Design review of the part built by this model. Coordinates are the model's own, in mm. A direction names the side the tool comes from. Give positions to 0.01 mm unless a question says otherwise; leave off trailing zeros. Loops run counter-clockwise (first coordinate to the right, second up) from the corner with the lowest first, then second, coordinate; pieces in that order, holes last. Notation, with made-up numbers: (-17.75, -17.5) - (-1.75, -17.5) arc R11 cw to (-1.75, -7.5) - close; hole circle Ø4 at (75.5, 35). An arc over 180 degrees is marked (long way). Write each question's results on one line, items separated by ' | '.
from build123d import *

# Parameters (mm, degrees)
SCHIZZO1_R                                           = 273.53258218
ESTRUSIONE_ESTRUSIONE1_DEPTH                         = 15
SCHIZZO5_R                                           = 273.53258218
ESTRUSIONE_ESTRUSIONE4_DEPTH                         = 685
SCHIZZO6_R                                           = 350
ESTRUSIONE_ESTRUSIONE5_DEPTH                         = 30
SMUSSO2_SIZE                                         = 20
FORO_LAMATO_PER_BULLONE_M20_A_TESTA_ESAG_D           = 22
FORO_LAMATO_PER_BULLONE_M20_A_TESTA_ESAG_CBORE_D     = 37.641
FORO_LAMATO_PER_BULLONE_M20_A_TESTA_ESAG_CBORE_DEPTH = 12.5
RIPETIZIONECIRCOLARE1_COUNT                          = 10
ESTRUSIONE_ESTRUSIONE6_START                         = 15
SCHIZZO10_R                                          = 9.25
ESTRUSIONE_ESTRUSIONE6_DEPTH                         = 15


with BuildPart() as part:
    # Schizzo1 → Estrusione-Estrusione1 (new body)
    with BuildSketch(Plane(origin=(0, 0, -132.207810149), x_dir=(-1, 0, 0), z_dir=(0, 0, -1))):
        with Locations(Location((214.171121607, -331.684921883, 0), (0, 0, 90))):
            Circle(SCHIZZO1_R)
        with BuildLine():
            ThreePointArc((-35.828878393, -322.434921883), (-45.078878393, -331.684921883), (-35.828878393, -340.934921883))
            ThreePointArc((-35.828878393, -340.934921883), (-26.578878393, -331.684921883), (-35.828878393, -322.434921883))
        make_face(mode=Mode.SUBTRACT)
        with BuildLine():
            ThreePointArc((-3.328878393, -340.934921883), (5.921121607, -331.684921883), (-3.328878393, -322.434921883))
            ThreePointArc((-3.328878393, -322.434921883), (-12.578878393, -331.684921883), (-3.328878393, -340.934921883))
        make_face(mode=Mode.SUBTRACT)
        with BuildLine():
            ThreePointArc((322.921121607, -134.074396559), (313.671121607, -143.324396559), (322.921121607, -152.574396559))
            ThreePointArc((322.921121607, -152.574396559), (332.171121607, -143.324396559), (322.921121607, -134.074396559))
        make_face(mode=Mode.SUBTRACT)
        with BuildLine():
            ThreePointArc((339.171121607, -124.428570936), (348.421121607, -115.178570936), (339.171121607, -105.928570936))
            ThreePointArc((339.171121607, -105.928570936), (329.921121607, -115.178570936), (339.171121607, -124.428570936))
        make_face(mode=Mode.SUBTRACT)
        with BuildLine():
            ThreePointArc((322.921121607, -529.295447206), (332.171121607, -520.045447206), (322.921121607, -510.795447206))
            ThreePointArc((322.921121607, -510.795447206), (313.671121607, -520.045447206), (322.921121607, -529.295447206))
        make_face(mode=Mode.SUBTRACT)
        with BuildLine():
            ThreePointArc((339.171121607, -557.441272829), (348.421121607, -548.191272829), (339.171121607, -538.941272829))
            ThreePointArc((339.171121607, -538.941272829), (329.921121607, -548.191272829), (339.171121607, -557.441272829))
        make_face(mode=Mode.SUBTRACT)
    extrude(amount=ESTRUSIONE_ESTRUSIONE1_DEPTH)

    # Schizzo5 → Estrusione-Estrusione4 (add)
    with BuildSketch(Plane(origin=(0, 0, -147.207810149), x_dir=(-1, 0, 0), z_dir=(0, 0, -1))):
        with Locations(Location((214.171121607, -331.684921883, 0), (0, 0, 90))):
            Circle(SCHIZZO5_R)
    extrude(amount=ESTRUSIONE_ESTRUSIONE4_DEPTH)

    # Schizzo6 → Estrusione-Estrusione5 (add)
    with BuildSketch(Plane(origin=(0, 0, -832.207810149), x_dir=(-1, 0, 0), z_dir=(0, 0, -1))):
        with Locations(Location((214.171121607, -331.684921883, 0), (0, 0, 90))):
            Circle(SCHIZZO6_R)
    extrude(amount=-ESTRUSIONE_ESTRUSIONE5_DEPTH)

    # Smusso2
    smusso2_edges = [part.edges().sort_by_distance(p)[0] for p in [
        (-214.171121607, -605.217504063, -802.207810149),
    ]]
    chamfer(smusso2_edges, length=SMUSSO2_SIZE)

    # Foro lamato per Bullone M20 a testa esagonale-1 (through all)
    with Locations(Plane(origin=(107.595169483, -331.684921883, -802.207810149), x_dir=(0, 1, 0), z_dir=(0, 0, 1))):
        with Locations((0, 0)):
            foro_lamato_per_bullone_m20_a_testa_esag = CounterBoreHole(FORO_LAMATO_PER_BULLONE_M20_A_TESTA_ESAG_D / 2, FORO_LAMATO_PER_BULLONE_M20_A_TESTA_ESAG_CBORE_D / 2, FORO_LAMATO_PER_BULLONE_M20_A_TESTA_ESAG_CBORE_DEPTH)

    # RipetizioneCircolare1: Foro lamato per Bullone M20 a testa esagonale-1 ×10 about axis
    ripetizionecircolare1_axis = Axis((-214.171121607, -331.684921883, 0), (0, 0, 1))
    for i in range(1, RIPETIZIONECIRCOLARE1_COUNT):
        add(foro_lamato_per_bullone_m20_a_testa_esag.rotate(ripetizionecircolare1_axis, i * 360 / RIPETIZIONECIRCOLARE1_COUNT), mode=Mode.SUBTRACT)

    # Schizzo10 → Estrusione-Estrusione6 (add)
    # profile 1 of 2: a face of its own
    with BuildSketch(Plane.XY.offset(-132.207810149).offset(ESTRUSIONE_ESTRUSIONE6_START)):
        with BuildLine():
            ThreePointArc((-339.171121607, -132.678570936), (-321.671121607, -115.178570936), (-339.171121607, -97.678570936))
            ThreePointArc((-339.171121607, -97.678570936), (-356.671121607, -115.178570936), (-339.171121607, -132.678570936))
        make_face()
        with Locations((-339.171121607, -115.178570936)):
            Circle(SCHIZZO10_R, mode=Mode.SUBTRACT)
    # profile 2 of 2: a face of its own
    with BuildSketch(Plane.XY.offset(-132.207810149).offset(ESTRUSIONE_ESTRUSIONE6_START)):
        with BuildLine():
            ThreePointArc((-339.171121607, -565.691272829), (-321.671121607, -548.191272829), (-339.171121607, -530.691272829))
            ThreePointArc((-339.171121607, -530.691272829), (-356.671121607, -548.191272829), (-339.171121607, -565.691272829))
        make_face()
        with Locations((-339.171121607, -548.191272829)):
            Circle(SCHIZZO10_R, mode=Mode.SUBTRACT)
    extrude(amount=-ESTRUSIONE_ESTRUSIONE6_DEPTH)

    # Smusso3: read off the stored shape, not the designer's step
    # Smusso3 outline → Smusso3 (revolve, cut)
    with BuildSketch(Plane(origin=(-339.171121607, -115.178570936, 0), x_dir=(1, 0, 0), z_dir=(0, -1, 0))):
        Polygon((17.5, -117.207810149), (15.5, -117.207810149), (17.5, -119.207810149), align=None)
    revolve(axis=Axis((-339.171121607, -115.178570936, 0), (0, 0, 1)), mode=Mode.SUBTRACT)

    # Smusso3 2 outline → Smusso3 2 (revolve, cut)
    with BuildSketch(Plane(origin=(-339.171121607, -548.191272829, 0), x_dir=(1, 0, 0), z_dir=(0, -1, 0))):
        Polygon((17.5, -117.207810149), (15.5, -117.207810149), (17.5, -119.207810149), align=None)
    revolve(axis=Axis((-339.171121607, -548.191272829, 0), (0, 0, 1)), mode=Mode.SUBTRACT)


solid = part.part
(1) Take a section at A-A on z = -679. Give the boundary of the cut face in (x, y).
Answers below:
outline: circle Ø547.07 at (-214.17, -331.68)
(2) Wall thickness on line 1 along Z through (x, y) = (7, -305.5); line 2 along Z through (x, y) = (-51, -625); line 3 along Y through (x, z) = (-402, -291): over which ranges is each line inside the solid? List them lowest first. Write a range as from..to.
Answers below:
line 1: -832.21..-132.21 | line 2: -832.21..-802.21 | line 3: -530.53..-132.84
(3) Draft analysis for pull direction Y (two halves, no side actions). For faces 1 (the cylindrical face through (22.376, -589.649, -817.418)), 2 (the flat face through (-486, -144, -814.708)), 3 (the flat face through (-446, -515, -802.208)), state which applies: pulls with the +Y half, pulls with the -Y half, needs draft (parallel to the pull), parting line crosses it, or undercut.
Answers below:
face 1: parting line crosses it | face 2: undercut | face 3: needs draft
(4) Tool access review of faces 4 (the cylindrical face through (-332.092, -142.12, -139.603)), 5 (the cylindrical face through (42.115, -152.791, -823.58)): name each direction out of +Z, -Z, +X, -X, +Y, -Y from which nothing blocks a thin tool from reaching the whole face with its end or side.
Answers below:
face 4: +Z | face 5: +Z, -Z
(5) Insertion check: P1, Ø19, axis at x = -475.5, y = -516, coming from the +Z side; P2, Ø8, axis at x = -364, z = -219, coming from the +Y side; P3, Ø8, axis at y = -216.5, z = -686.5, coming from the -X side; P4, Ø17.5, axis at x = 46.14, y = -142.56, coming from the -Z side. Each pin has a flat end and moves straight along its axis. Give the tip position at first contact, or say it passes through.
Answers below:
P1: z = -814.71 | P2: y = -100.27 | P3: x = -464.09 | P4: through
